```python
from build123d import *

# Parameters (mm, degrees)
F0_W        = 12.7
F0_H        = 25.4
F1_DEPTH    = 9.525
F2_T1_DEPTH = 50.8
F2_T3_DEPTH = 50.8
F3_R        = 3.175
F4_DEPTH    = 101.601
F5_W        = 40.64
F5_H        = 7.62
F6_DEPTH    = 101.601
F7_R        = 5.07999


# Not quite as in the source:
# - a fillet or chamfer that OpenCascade refuses, or shapes differently, is made with other operations: its cross-section is extruded or revolved along the edge and cut away or added
# - a fillet or chamfer is up to 0.001 mm smaller than in the source, because OpenCascade refuses the exact size


with BuildPart() as f1:
    # F0 (on Front) → F1 (new body)
    with BuildSketch(Plane.XZ):
        with Locations((19.05, 38.1)):
            Rectangle(F0_W, F0_H)
        Polygon((12.7, 25.4), (12.7, 50.8), (-25.4, 50.8), (-25.4, -50.8), (12.7, -50.8), (12.7, -25.4), (12.7, 0), align=None)
        with Locations((19.05, -12.7)):
            Rectangle(F0_W, F0_H)
    extrude(amount=F1_DEPTH)

    # F2: fillet of radius 5.08 on 4 edges, made by hand

    # F2_s2 → F2_t1 (cut)
    with BuildSketch(Plane.XY.offset(12.7)):
        with BuildLine():
            ThreePointArc((25.4, -5.08), (23.9121024484, -1.4878975516), (20.32, 0))
            Line((20.32, 0), (25.4, 0))
            Line((25.4, 0), (25.4, -5.08))
        make_face()
        with BuildLine():
            ThreePointArc((25.4, -4.445), (23.9121024484, -8.0371024484), (20.32, -9.525))
            Line((20.32, -9.525), (25.4, -9.525))
            Line((25.4, -9.525), (25.4, -4.445))
        make_face()
    extrude(amount=F2_T1_DEPTH, mode=Mode.SUBTRACT)

    # F2_s4 → F2_t3 (cut)
    with BuildSketch(Plane.XY.offset(-38.1)):
        with BuildLine():
            ThreePointArc((25.4, -5.08), (23.9121024484, -1.4878975516), (20.32, 0))
            Line((20.32, 0), (25.4, 0))
            Line((25.4, 0), (25.4, -5.08))
        make_face()
        with BuildLine():
            ThreePointArc((25.4, -4.445), (23.9121024484, -8.0371024484), (20.32, -9.525))
            Line((20.32, -9.525), (25.4, -9.525))
            Line((25.4, -9.525), (25.4, -4.445))
        make_face()
    extrude(amount=F2_T3_DEPTH, mode=Mode.SUBTRACT)

    # F3 (on face) → F4 (cut, through all)
    with BuildSketch(Plane.XY.offset(50.8)):
        with Locations((20.32, -4.7625)):
            Circle(F3_R)
    extrude(amount=-F4_DEPTH, mode=Mode.SUBTRACT)

    # F5 (on face) → F6 (cut, through all)
    with BuildSketch(Plane.XY.offset(50.8)):
        with Locations((-5.08, -3.81)):
            Rectangle(F5_W, F5_H)
    extrude(amount=-F6_DEPTH, mode=Mode.SUBTRACT)

    # F7 (radius 5.08 in the source; OpenCascade refuses exactly that, so slightly less here)
    f7_edges = [f1.edges().sort_by_distance(p)[0] for p in [
        (15.24, 0, 38.1),
        (15.24, 0, -12.7),
    ]]
    fillet(f7_edges, radius=F7_R)


solid = f1.part
```
Geometry check sheet. Reference: the model listing, model coordinates, mm. A direction names the side the tool comes from. Give positions to 0.01 mm unless a question says otherwise; leave off trailing zeros. Order: outer loops, then holes, each group sorted by start corner. A loop starts at its lowest first (then second) coordinate and runs counter-clockwise, first axis right, second up. Notation, with made-up numbers: (47, -35.75) -> (91, -35.75) arc R18 cw to (91, -6.75) -> close; hole circle Ø7 at (-1, 19). An arc over 180 degrees is marked (long way). Write each question's results on one line, items separated by ' | '. Start each with the question number.
(1) Scan lines: line 1 (Y direction, x = 20, z = 36) (3 decimals); line 2 (Z direction, x = 19, y = -1.75); line 3 (Y direction, x = -9.5, z = -32.5) (3 decimals). Record each from-to range of solid material in increasing order.
(2) Sectioned sample at A-A (y = -3). Enter the section's corners in (x, z).
(3) Gauge pin test, flat ends, axial feed: P1, Ø1, axis at y = -9, z = 16.5, coming from the +X side; P2, Ø4, axis at y = -2, z = -1.5, coming from the -X side; P3, Ø0.8, axis at y = -6.5, z = -12, coming from the -X side. Record the tip position at first contact, or that the pin passes through.
(4) Sectioned sample at D-D (x = -8). Enter the section's corners in (y, z) (3 decimals), plus the area to 3 significant figures.
(5) Access from +Z, -Z, +X, -X, +Y, -Y to the whole of each face (thin tool, end or side, straight path). Record for faces 1 (the face through (12.7, -9, 13)), 2 (the face through (17.15, -4.62, -12.52)), 3 (the face through (15.24, -6, 38)), 4 (the face through (12.7, -9, -38)), 5 (the face through (6, -8, 50.8)).
(6) Mould release check, pull along Z, two halves, no side actions. Record for faces 6 (the face through (-7, -9, -50.8)), 7 (the face through (17.5, -6.8, 25.4)), 8 (the face through (23.84, -8.11, 37.92)): pulls with the +Z half, pulls with the -Z half, needs draft (parallel to the pull), parting line crosses it, or undercut.
(7) Sectioned sample at C-C (z = 8). Enter the section's corners in (x, y) (3 decimals), plus the area to 3 significant figures.
Answer below:
1) line 1: -9.525 to -7.921, -1.604 to -0.01 | line 2: -25.4 to 0, 25.4 to 50.8 | line 3: -9.525 to -7.62
2) outline: (15.69, -25.4) -> (17.68, -25.4) -> (17.68, 0) -> (15.69, 0) -> close; (15.69, 25.4) -> (17.68, 25.4) -> (17.68, 50.8) -> (15.69, 50.8) -> close; (22.96, -25.4) -> (24.95, -25.4) -> (24.95, 0) -> (22.96, 0) -> close; (22.96, 25.4) -> (24.95, 25.4) -> (24.95, 50.8) -> (22.96, 50.8) -> close
3) P1: x = 12.7 | P2: x = 15.36 | P3: x = 15.24
4) outline: (-9.525, -50.8) -> (-7.62, -50.8) -> (-7.62, 50.8) -> (-9.525, 50.8) -> close | area: 194 mm2
5) face 1: +X, +Y, -Y | face 2: +Z, -Z | face 3: +Z, -Z, -X, +Y | face 4: -Z, +X, +Y, -Y | face 5: +Z, +X, -X, +Y, -Y
6) face 6: pulls with the -Z half | face 7: undercut | face 8: needs draft
7) outline: (-25.4, -9.525) -> (12.7, -9.525) -> (12.7, -7.62) -> (-25.4, -7.62) -> close | area: 72.6 mm2
